Autodesk Inventor part; units mm, degrees
ref_plane "YZ Plane" through (0, 0, 0) normal (1, 0, 0) x (0, 1, 0)
ref_plane "XZ Plane" through (0, 0, 0) normal (0, 1, 0) x (-1, 0, 0)
ref_plane "XY Plane" through (0, 0, 0) normal (0, 0, 1) x (1, 0, 0)
sketch "Sketch1" plane through (0, 0, 0) normal (0, 0, 1) x (1, 0, 0)
  line L0 (0, 0) -> (43, 0)
  line L1 (43, 0) -> (43, 15)
  line L2 (43, 15) -> (0, 15)
  line L3 (0, 15) -> (0, 0)
  dimension "d0" = 43
  dimension "d1" = 15
extrude "Extrusion1" add sketch "Sketch1" along normal blind 5
sketch "Sketch2" plane through (0, 15, 0) normal (0, 1, 0) x (1, 0, 0)
  point P0 (0, 0)
sketch "Sketch3" plane through (0, 15, 0) normal (0, 1, 0) x (1, 0, 0)
  line L0 (1.8425, -12.4637) -> (1.8425, -4.1304)
  line L1 (1.8425, -4.1304) -> (2.9382, -4.1304)
  line L2 (2.9382, -4.1304) -> (2.9382, -12.4637)
  line L3 (2.9382, -12.4637) -> (1.8425, -12.4637)
  line L4 (1.8425, -12.4637) -> (1.8425, -4.1304)
  line L5 (7.4078, -4.1304) -> (8.3192, -4.1304)
  line L6 (8.3192, -4.1304) -> (8.3192, -12.4637)
  line L7 (8.3192, -12.4637) -> (7.4078, -12.4637)
  line L8 (7.4078, -12.4637) -> (7.4078, -4.1304)
  line L9 (12.7537, -4.1304) -> (13.7002, -4.1304)
  line L10 (13.7002, -4.1304) -> (13.7002, -12.4637)
  line L11 (13.7002, -12.4637) -> (12.7537, -12.4637)
  line L12 (12.7537, -12.4637) -> (12.7537, -4.1304)
  line L13 (18.7833, -4.1304) -> (19.7298, -4.1304)
  line L14 (19.7298, -4.1304) -> (19.7298, -12.4637)
  line L15 (19.7298, -12.4637) -> (18.7833, -12.4637)
  line L16 (18.7833, -12.4637) -> (18.7833, -4.1304)
  line L17 (24.6292, -4.1304) -> (25.5788, -4.1304)
  line L18 (25.5788, -4.1304) -> (25.5788, -12.4637)
  line L19 (25.5788, -12.4637) -> (24.6292, -12.4637)
  line L20 (24.6292, -12.4637) -> (24.6292, -4.1304)
  line L21 (30.4626, -4.1304) -> (31.367, -4.1304)
  line L22 (31.367, -4.1304) -> (31.367, -12.4637)
  line L23 (31.367, -12.4637) -> (30.4626, -12.4637)
  line L24 (30.4626, -12.4637) -> (30.4626, -4.1304)
  line L25 (36.1151, -4.1304) -> (37.11, -4.1304)
  line L26 (37.11, -4.1304) -> (37.11, -12.4637)
  line L27 (37.11, -12.4637) -> (36.1151, -12.4637)
  line L28 (36.1151, -12.4637) -> (36.1151, -4.1304)
  line L29 (40.4111, -4.1304) -> (41.3607, -4.1304)
  line L30 (41.3607, -4.1304) -> (41.3607, -12.4637)
  line L31 (41.3607, -12.4637) -> (40.4111, -12.4637)
  line L32 (40.4111, -12.4637) -> (40.4111, -4.1304)
  line L33 (1.8425, -4.1304) -> (2.9382, -4.1304)
  line L34 (7.4078, -4.1304) -> (8.3192, -4.1304)
  line L35 (12.7537, -4.1304) -> (13.7002, -4.1304)
  line L36 (18.7833, -4.1304) -> (19.7298, -4.1304)
  line L37 (24.6292, -4.1304) -> (25.5788, -4.1304)
  line L38 (30.4626, -4.1304) -> (31.367, -4.1304)
  line L39 (36.1151, -4.1304) -> (37.11, -4.1304)
  line L40 (40.4111, -4.1304) -> (41.3607, -4.1304)
  line L41 (41.3607, -12.4637) -> (40.4111, -12.4637)
  line L42 (37.11, -12.4637) -> (36.1151, -12.4637)
  line L43 (31.367, -12.4637) -> (30.4626, -12.4637)
  line L44 (25.5788, -12.4637) -> (24.6292, -12.4637)
  line L45 (19.7298, -12.4637) -> (18.7833, -12.4637)
  line L46 (13.7002, -12.4637) -> (12.7537, -12.4637)
  line L47 (8.3192, -12.4637) -> (7.4078, -12.4637)
  line L48 (2.9382, -12.4637) -> (1.8425, -12.4637)
  point P0 (0, 0)
extrude "Extrusion2" add sketch "Sketch3" along normal blind 1
sketch "Sketch4" plane through (0, 0, 0) normal (0, -1, 0) x (1, 0, 0)
  line L0 (41.3607, 4.1304) -> (40.4111, 4.1304)
  line L1 (40.4111, 4.1304) -> (40.4111, 12.4637)
  line L2 (41.3607, 4.1304) -> (40.4111, 4.1304)
  line L3 (40.4111, 4.1304) -> (40.4111, 12.4637)
  line L4 (40.4111, 12.4637) -> (41.3607, 12.4637)
  line L5 (41.3607, 12.4637) -> (41.3607, 4.1304)
  line L6 (36.1151, 4.1304) -> (37.11, 4.1304)
  line L7 (36.1151, 5) -> (36.1151, 12.4637)
  line L8 (37.11, 4.1304) -> (36.1151, 4.1304)
  line L9 (36.1151, 4.1304) -> (36.1151, 12.4637)
  line L10 (36.1151, 12.4637) -> (37.11, 12.4637)
  line L11 (37.11, 12.4637) -> (37.11, 4.1304)
  line L12 (30.4626, 4.1304) -> (30.4626, 12.4637)
  line L13 (31.367, 4.1304) -> (30.4626, 4.1304)
  line L14 (30.4626, 4.1304) -> (30.4626, 12.4637)
  line L15 (30.4626, 12.4637) -> (31.367, 12.4637)
  line L16 (31.367, 12.4637) -> (31.367, 4.1304)
  line L17 (25.5788, 4.1304) -> (24.6292, 4.1304)
  line L18 (24.6292, 4.1304) -> (24.6292, 12.4637)
  line L19 (25.5788, 4.1304) -> (24.6292, 4.1304)
  line L20 (24.6292, 4.1304) -> (24.6292, 12.4637)
  line L21 (24.6292, 12.4637) -> (25.5788, 12.4637)
  line L22 (25.5788, 12.4637) -> (25.5788, 4.1304)
  line L23 (19.7298, 12.4637) -> (19.7298, 4.1304)
  line L24 (18.7833, 4.1304) -> (18.7833, 12.4637)
  line L25 (19.7298, 4.1304) -> (18.7833, 4.1304)
  line L26 (18.7833, 4.1304) -> (18.7833, 12.4637)
  line L27 (18.7833, 12.4637) -> (19.7298, 12.4637)
  line L28 (19.7298, 12.4637) -> (19.7298, 4.1304)
  line L29 (13.7002, 4.1304) -> (13.7002, 5)
  line L30 (12.7537, 4.1304) -> (12.7537, 12.4637)
  line L31 (13.7002, 4.1304) -> (12.7537, 4.1304)
  line L32 (12.7537, 4.1304) -> (12.7537, 12.4637)
  line L33 (12.7537, 12.4637) -> (13.7002, 12.4637)
  line L34 (13.7002, 12.4637) -> (13.7002, 4.1304)
  line L35 (8.3192, 4.1304) -> (8.3192, 5)
  line L36 (7.4078, 4.1304) -> (7.4078, 12.4637)
  line L37 (8.3192, 4.1304) -> (7.4078, 4.1304)
  line L38 (7.4078, 4.1304) -> (7.4078, 12.4637)
  line L39 (7.4078, 12.4637) -> (8.3192, 12.4637)
  line L40 (8.3192, 12.4637) -> (8.3192, 4.1304)
  line L41 (2.9382, 4.1304) -> (1.8425, 4.1304)
  line L42 (1.8425, 4.1304) -> (1.8425, 12.4637)
  line L43 (2.9382, 4.1304) -> (1.8425, 4.1304)
  line L44 (1.8425, 4.1304) -> (1.8425, 12.4637)
  line L45 (1.8425, 12.4637) -> (2.9382, 12.4637)
  line L46 (2.9382, 12.4637) -> (2.9382, 4.1304)
  point P0 (0, 0)
extrude "Extrusion3" add sketch "Sketch4" along normal blind 1
properties part number "hbridge"
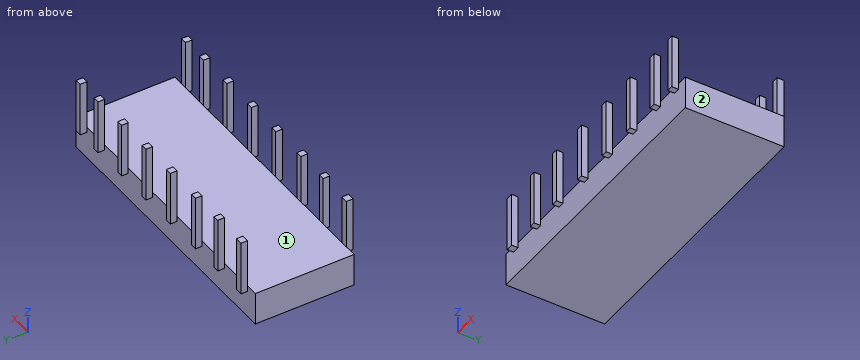
Verification items for the finished model (mm, model axes). Face numbers are marked on the shaded views. Give positions to 0.01 mm unless a question says otherwise; leave off trailing zeros. Loops run counter-clockwise (first coordinate to the right, second up) from the corner with the lowest first, then second, coordinate; pieces in that order, holes last. Notation, with made-up numbers: M -13.5,79 L 12.5,79 A17 ccw 12.5,101 Z; hole C 88.5,77 d9. An arc over 180 degrees is marked long. Return JSON: item names as keys, results as strings.
1) Gauge pin test, flat ends, axial feed: P1, Ø3, axis at x = 25.5, y = 6, coming from the +Z side; P2, Ø1.1, axis at y = 15.5, z = 10, coming from the -X side; P3, Ø1.1, axis at y = -0.5, z = 8, coming from the +X side; P4, Ø6, axis at x = 7, z = 6.5, coming from the +Y side. Record the tip position at first contact, or that the pin passes through.
Findings:
{"P1": "stops at z = 5", "P2": "stops at x = 1.84", "P3": "stops at x = 41.36", "P4": "stops at y = 16"}
2) Mould release check, pull along Y, two halves, no side actions. Record for the marked faces 1 and 2: released by +Y, released by -Y, zero draft, split by the parting line, or undercut.
Findings:
{"face 1": "undercut", "face 2": "zero draft"}
3) Section check C-C, the plane y = 2.5. Enter the section's corners in (x, z).
Findings:
{"outline": "M 0,0 L 43,0 L 43,5 L 0,5 Z"}
4) Section check A-A, the plane z = 8.5. Count the separate pieces of the cut face and the enclosed holes in it, and give its area (3 significant figures).
Findings:
{"separate pieces": "16", "enclosed holes": "0", "area": "15.4 mm2"}
5) Section check B-B, the plane x = 11. Enter the section's corners in (y, z), and give its area (3 significant figures).
Findings:
{"outline": "M 0,0 L 15,0 L 15,5 L 0,5 Z", "area": "75.0 mm2"}
6) Material ranges on L1, parallel to Y at x = 36.5, z = 12; L2, parallel to Z at x = 7.5, y = 4.5; L3, parallel to Y at x = 7.5, z = 3.75, recorded low to high. Write a range as [from, to].
Findings:
{"L1": "y = [-1, 0], [15, 16]", "L2": "z = [0, 5]", "L3": "y = [0, 15]"}
